Part model, mm, in its own coordinate system. Coordinates: 2 decimals unless noted, no trailing zeros. Use a Markdown table: item, result. Add a question column.
Q1. Slice it at A-A on y = 0. Count the separate pieces of the cut face and the enclosed holes in it, then the cut area to 3 significant figures.
Q2. Wall check: L1, parallel to Y at x = 0, z = 17.75; L2, parallel to X at y = -26.5, z = 4.5; L3, parallel to X at y = -40.5, z = 11.25. Give the ranges that are in metal, low to high. Write a range as from..to.
Q3. Pin check, flat tips, straight feed: pin 1 Ø5 at (y, z) = (-24, 5.5) entering from +X; pin 2 Ø1.5 at (x, z) = (35, 17.5) entering from +Y; pin 3 Ø8 at (x, z) = (-34, 7) entering from -Y; pin 4 Ø1 at (x, z) = (9, 3.5) entering from -Y. Stop position of each tip, or through.
Q4. Mould opens along X. For faces 1 (the flat face through (-44.77, -49.01, 12.56)), 2 (the cylindrical face through (-2.579, -1.978, 12.325)) say: released by +X, released by -X, zero draft, split by the parting line, or undercut.
from build123d import *

# Parameters (mm, degrees)
SKETCH_1_R               = 3.25
EXTRUDE_1_DEPTH          = 25
CUT_EXTRUDE_1_DEPTH      = 82.79550394
CUT_EXTRUDE_1_DEPTH_BACK = 82.79550394


with BuildPart() as part:
    # 草圖1 → 填料-伸長1 (new body)
    with BuildSketch(Plane.XY):
        with BuildLine():
            Line((-41, -60), (-40, -60))
            add(Edge.make_bspline(
                [(-44, -6), (-55, -25), (-40, -60)],
                knots=[0, 0, 0, 1, 1, 1], degree=2))
            add(Edge.make_bspline(
                [(-6.5, 2), (-31.607950909, -0.616387712), (-44, -6)],
                knots=[0, 0, 0, 1, 1, 1], degree=2))
            add(Edge.make_bspline(
                [(-6.5, 2), (0, -12), (6.5, 2)],
                knots=[0, 0, 0, 1, 1, 1], degree=2))
            add(Edge.make_bspline(
                [(6.5, 2), (32.228671013, -0.616387712), (44, -6)],
                knots=[0, 0, 0, 1, 1, 1], degree=2))
            add(Edge.make_bspline(
                [(44, -6), (55, -25), (40, -60)],
                knots=[0, 0, 0, 1, 1, 1], degree=2))
            Line((40, -60), (41, -60))
            add(Edge.make_bspline(
                [(45, -5), (56, -25), (41, -60)],
                knots=[0, 0, 0, 1, 1, 1], degree=2))
            add(Edge.make_bspline(
                [(-45, -5), (0, 13), (45, -5)],
                knots=[0, 0, 0, 1, 1, 1], degree=2))
            add(Edge.make_bspline(
                [(-45, -5), (-56, -25), (-41, -60)],
                knots=[0, 0, 0, 1, 1, 1], degree=2))
        make_face()
        Circle(SKETCH_1_R, mode=Mode.SUBTRACT)
    extrude(amount=EXTRUDE_1_DEPTH)

    # 草圖2 → 除料-伸長1 (cut, two sides: drawn at the far end of the back side and taken through both)
    with BuildSketch(Plane(origin=(0, 0, 0), x_dir=(0, 0, -1), z_dir=(1, 0, 0)).offset(-CUT_EXTRUDE_1_DEPTH_BACK)):
        Polygon((-28.906277967, -52.492311819), (4.067188518, -45.468378129), (5.936036077, -63.083878207), (-26.90117602, -70.571484262), (-30.384906988, -68.381487837), align=None)
    extrude(amount=CUT_EXTRUDE_1_DEPTH + CUT_EXTRUDE_1_DEPTH_BACK, mode=Mode.SUBTRACT)


solid = part.part
Recorded:
| question | item | result |
|---|---|---|
| 1 | separate pieces | 4 |
| 1 | enclosed holes | 0 |
| 1 | area | 529 mm² |
| 2 | L1 | -5..-3.25, 3.25..4 |
| 2 | L2 | -49.62..-48.63, 48.63..49.62 |
| 2 | L3 | -47.62..-46.65, 46.65..47.62 |
| 3 | pin 1 | x = 49.65 |
| 3 | pin 2 | y = -1.21 |
| 3 | pin 3 | y = -3.79 |
| 3 | pin 4 | y = 1.68 |
| 4 | face 1 | zero draft |
| 4 | face 2 | undercut |
